```python
from build123d import *

# Parameters (mm, degrees)
BOX005_W     = 42
BOX005_H     = 8
BOX005_DEPTH = 2
BOX004_W     = 42
BOX004_H     = 44
BOX004_DEPTH = 2
BOX001_W     = 2
BOX001_H     = 44
BOX001_DEPTH = 44
BOX002_W     = 2
BOX002_H     = 44
BOX002_DEPTH = 44
BOX003_W     = 2
BOX003_H     = 44
BOX003_DEPTH = 44
BOX_W        = 2
BOX_H        = 44
BOX_DEPTH    = 44


with BuildPart() as cubo005:
    # Box005 → Box005 (new body)
    with BuildSketch(Plane(origin=(2, 18, 42), x_dir=(1, 0, 0), z_dir=(0, 0, 1))):
        with Locations((21, 4)):
            Rectangle(BOX005_W, BOX005_H)
    extrude(amount=BOX005_DEPTH)


with BuildPart() as cut:
    # Box004 → Box004 (new body)
    with BuildSketch(Plane(origin=(2, 0, 42), x_dir=(1, 0, 0), z_dir=(0, 0, 1))):
        with Locations((21, 22)):
            Rectangle(BOX004_W, BOX004_H)
    extrude(amount=BOX004_DEPTH)

    # Cut: cut Cubo005
    add(cubo005.part, mode=Mode.SUBTRACT)


with BuildPart() as cubo001:
    # Box001 → Box001 (new body)
    with BuildSketch(Plane(origin=(0, 0, 0), x_dir=(0, -1, 0), z_dir=(0, 0, 1))):
        with Locations((1, 22)):
            Rectangle(BOX001_W, BOX001_H)
    extrude(amount=BOX001_DEPTH)


with BuildPart() as cubo002:
    # Box002 → Box002 (new body)
    with BuildSketch(Plane(origin=(0, 46, 0), x_dir=(0, -1, 0), z_dir=(0, 0, 1))):
        with Locations((1, 22)):
            Rectangle(BOX002_W, BOX002_H)
    extrude(amount=BOX002_DEPTH)


with BuildPart() as cubo003:
    # Box003 → Box003 (new body)
    with BuildSketch(Plane(origin=(0, 0, 0), x_dir=(0, 0, -1), z_dir=(1, 0, 0))):
        with Locations((1, 22)):
            Rectangle(BOX003_W, BOX003_H)
    extrude(amount=BOX003_DEPTH)


with BuildPart() as fusion002:
    # Box → Box (new body)
    with BuildSketch(Plane.XY):
        with Locations((1, 22)):
            Rectangle(BOX_W, BOX_H)
    extrude(amount=BOX_DEPTH)

    # Fusion: union Cubo001, Cubo002, Cubo003
    add(cubo001.part)
    add(cubo002.part)
    add(cubo003.part)

    # Fusion002: union Cut
    add(cut.part)


solid = fusion002.part
```
Could you check a few things on this model? Use its own coordinates, in mm. A direction names the side the tool comes from. Give positions to 0.01 mm unless a question says otherwise; leave off trailing zeros. Write each loop counter-clockwise with the first axis right and the second up, starting at its lowest first coordinate (ties: lowest second). Pieces come first, ordered by that corner, then holes. Notation, with made-up numbers: (78.5, -3.5) - (109.5, -3.5) arc R16 cw to (109.5, 9.5) - close; hole circle Ø3 at (67, 6.5). An arc over 180 degrees is marked (long way). One line per item, written item: value. Start each with the question number.
Item 1: Please list where these lines run through material, in increasing order: line 1 (Y direction, x = 9, z = 8); line 2 (Z direction, x = 25, y = 35); line 3 (Z direction, x = 11.5, y = 25). Write a range as from..to.
Item 2: Which directions (+Z, -Z, +X, -X, +Y, -Y) give clear straight access to the entire face, cutting with the end or side of a thin tool? Please do faces 5 (the face through (23, 0, 21)), 6 (the face through (22, 45, 0)), 7 (the face through (22, -1, 0)), 8 (the face through (23, 18, 43)).
Item 3: Imagine slicing it at B-B, the plane y = 28. List the corners of the cut face in (x, z) for me.
Item 4: I'm going to push flat-ended pins straight in: pin 1 (1 mm diameter, centred on x = 11.5, z = -1, fed in from +Y); pin 2 (1 mm diameter, centred on y = 39.5, z = 35, fed in from +X); pin 3 (1 mm diameter, centred on x = 32.5, z = -1, fed in from -Y). Where does each tip first touch, or does it pass through?
Item 5: Imagine slicing it at C-C, the plane z = 3. List the corners of the cut face in (x, y) for me, and give its area (3 significant figures).
Item 6: If we mould it in two halves opening along Y, with no side actions, what happens to faces 1 (the face through (22, -2, 22)), 2 (the face through (44, 22, -1)), 3 (the face through (23, 44, 21)), 4 (the face through (22, 44, -1))? For each: +Y half, -Y half, draft (parallel to the pull), parting line (faces both ways), or undercut.
Geometry says:
1. line 1: -2..0, 44..46
1. line 2: -2..0, 42..44
1. line 3: -2..0
2. face 5: +X
2. face 6: -Z, +X, -X, +Y
2. face 7: -Z, +X, -X, -Y
2. face 8: +Z, +X
3. outline: (0, -2) - (44, -2) - (44, 0) - (2, 0) - (2, 42) - (44, 42) - (44, 44) - (0, 44) - close
4. pin 1: y = 44
4. pin 2: x = 2
4. pin 3: y = 0
5. outline: (0, -2) - (44, -2) - (44, 0) - (2, 0) - (2, 44) - (44, 44) - (44, 46) - (0, 46) - close
5. area: 264 mm^2
6. face 1: -Y half
6. face 2: draft
6. face 3: undercut
6. face 4: +Y half
